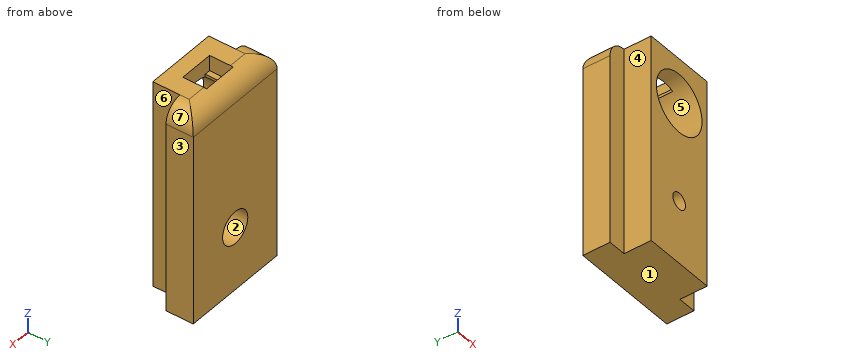
from build123d import *

# Parameters (mm, degrees)
SKETCH1_W           = 12
SKETCH1_H           = 23
BOSS_EXTRUDE1_DEPTH = 6
SKETCH2_W           = 2
SKETCH2_H           = 3
CUT_EXTRUDE1_DEPTH  = 25.515301344
SKETCH3_W           = 3.82
SKETCH3_H           = 2.6
CUT_EXTRUDE2_DEPTH  = 1.71
SKETCH4_W           = 2.566615902
SKETCH4_H           = 2.2
CUT_EXTRUDE3_DEPTH  = 3.1
CUT_EXTRUDE4_REACH  = 16.292
SKETCH5_R           = 3.265
FILLET1_R           = 2


with BuildPart() as part:
    # Sketch1 → Boss-Extrude1 (new body)
    with BuildSketch(Plane(origin=(0, 0, 0), x_dir=(1, 0, 0), z_dir=(0, 1, 0))):
        Rectangle(SKETCH1_W, SKETCH1_H)
    extrude(amount=BOSS_EXTRUDE1_DEPTH)

    # Sketch2 → Cut-Extrude1 (cut, through all)
    with BuildSketch(Plane.XY.offset(11.5)):
        with Locations((5, 1.5)):
            Rectangle(SKETCH2_W, SKETCH2_H)
        with Locations((-5, 1.5)):
            Rectangle(SKETCH2_W, SKETCH2_H)
    extrude(amount=-CUT_EXTRUDE1_DEPTH, mode=Mode.SUBTRACT)

    # Sketch3 → Cut-Extrude2 (cut)
    with BuildSketch(Plane.XY.offset(11.5)):
        with Locations((0, 3)):
            Rectangle(SKETCH3_W, SKETCH3_H)
    extrude(amount=-CUT_EXTRUDE2_DEPTH, mode=Mode.SUBTRACT)

    # Sketch4 → Cut-Extrude3 (cut)
    with BuildSketch(Plane.XY.offset(9.79)):
        with Locations((0, 2.8)):
            Rectangle(SKETCH4_W, SKETCH4_H)
    extrude(amount=-CUT_EXTRUDE3_DEPTH, mode=Mode.SUBTRACT)

    # Cut-Extrude4: up to this face of the body (flat: up to its plane)
    cut_extrude4_end = Plane(part.part.faces().sort_by_distance((0, 3.9, 8.24))[0])
    # Sketch5 → Cut-Extrude4 (cut, up to the picked face)
    with BuildSketch(Plane.XZ, mode=Mode.PRIVATE) as cut_extrude4_sk1:
        with Locations(Location((0, 6.5, 0), (0, 0, 270))):
            Circle(SKETCH5_R)
    cut_extrude4_tool1 = split(extrude(cut_extrude4_sk1.sketch, amount=-CUT_EXTRUDE4_REACH, mode=Mode.PRIVATE), bisect_by=cut_extrude4_end, keep=Keep.BOTH, mode=Mode.PRIVATE)
    add(cut_extrude4_tool1.solids().sort_by(Axis((0, 0, 6.5), (0, 1, 0)))[0], mode=Mode.SUBTRACT)

    # Fillet1
    # the kernel refuses this fillet: 2 mm, written as the material it takes off along each edge
    with BuildSketch(Plane(origin=(6, -2, 11.5), x_dir=(0, 0, -1), z_dir=(0, 1, 0))) as fillet1_piece_1:
        with BuildLine():
            CenterArc((FILLET1_R, FILLET1_R), FILLET1_R, 180, 90)
            Line((0, FILLET1_R), (0, 0))
            Line((0, 0), (FILLET1_R, 0))
        make_face()
    extrude(amount=13, mode=Mode.SUBTRACT)
    with BuildSketch(Plane(origin=(-11, 6, 11.5), x_dir=(0, 0, -1), z_dir=(1, 0, 0))) as fillet1_piece_2:
        with BuildLine():
            CenterArc((FILLET1_R, -FILLET1_R), FILLET1_R, 90, 90)
            Line((0, -FILLET1_R), (0, 0))
            Line((0, 0), (FILLET1_R, 0))
        make_face()
    extrude(amount=22, mode=Mode.SUBTRACT)
    with BuildSketch(Plane(origin=(-6, -2, 11.5), x_dir=(0, 0, -1), z_dir=(0, 1, 0))) as fillet1_piece_3:
        with BuildLine():
            CenterArc((FILLET1_R, -FILLET1_R), FILLET1_R, 90, 90)
            Line((0, -FILLET1_R), (0, 0))
            Line((0, 0), (FILLET1_R, 0))
        make_face()
    extrude(amount=13, mode=Mode.SUBTRACT)

    # Sketch7 → CSK SLOT for M1.6 Countersunk Flat Head Screw1 (revolve, cut)
    with BuildSketch(Plane(origin=(0, 6, -4.5), x_dir=(0, 0, 1), z_dir=(1, 0, 0))):
        Polygon((0, 0), (0, 6), (0.9, 6), (0.9, 4.9), (1.8, 4), (1.8, 0), align=None)
    revolve(axis=Axis((0, 12.35, -4.5), (0, -1, 0)), mode=Mode.SUBTRACT)


solid = part.part
Part model, mm, in its own coordinate system. Face numbers are marked on the shaded views. A direction names the side the tool comes from. Give positions to 0.01 mm unless a question says otherwise; leave off trailing zeros. Write each loop counter-clockwise with the first axis right and the second up, starting at its lowest first coordinate (ties: lowest second). Pieces come first, ordered by that corner, then holes.
1) Cut at A-A on z = -4.5. Write the cut outline in (x, y).
Resolved:
outline: (-6, 3) - (-4, 3) - (-4, 0) - (-0.9, 0) - (-0.9, 1.1) - (-1.8, 2) - (-1.8, 6) - (-6, 6) - close; (0.9, 0) - (4, 0) - (4, 3) - (6, 3) - (6, 6) - (1.8, 6) - (1.8, 2) - (0.9, 1.1) - close
2) Cut at B-B on x = 0. Write the cut outline in (y, z) (3 decimals), then the cut area to 3 significant figures.
Resolved:
outline: (0, -11.5) - (6, -11.5) - (6, -6.3) - (2, -6.3) - (1.1, -5.4) - (0, -5.4) - close; (0, -3.6) - (1.1, -3.6) - (2, -2.7) - (6, -2.7) - (6, 9.5) arc R2 ccw to (4.3, 11.477) - (4.3, 9.79) - (3.9, 9.79) - (3.9, 3.235) - (0, 3.235) - close; (0, 9.765) - (1.7, 9.765) - (1.7, 11.5) - (0, 11.5) - close
area: 88.4 mm2
3) Cut at D-D on y = 1.4. Write the cut outline in (x, z) (3 decimals).
Resolved:
outline: (-4, -11.5) - (4, -11.5) - (4, 11.5) - (-4, 11.5) - close; hole circle Ø6.53 at (0, 6.5); hole circle Ø2.4 at (0, -4.5)
4) Which spindle directions (+Z, -Z, +X, -X, +Y, -Y) get a long thin tool onto all of the face, cutting with end or side? Do the marked faces 4, 5, 6 and 7. Say none if no direction does.
Resolved:
face 4: +Z, -Z, -X, -Y
face 5: -Y
face 6: +Z, -Z, +X, -Y
face 7: +Z, +X, +Y, -Y
5) Pin check, flat tips, straight feed: pin 1 (0.5 mm diameter, centred on y = 2.5, z = 10.5, fed in from +X); pin 2 (1.4 mm diameter, centred on y = 3.5, z = 10.5, fed in from -X); pin 3 (0.6 mm diameter, centred on x = 0.5, z = 11, fed in from +Y). Stop position of each tip, or through.
Resolved:
pin 1: stops at x = 4
pin 2: stops at x = -5.98
pin 3: stops at y = 5.6
6) Probe L1, parallel to X at y = 2.9, z = 6.5 (3 decimals); L2, parallel to Z at x = 0, y = 0.4 (3 decimals); L3, parallel to Z at x = 0, y = 4.1. List the from-to ranges inside material, lowest first.
Resolved:
L1: x = -4 to -3.265, 3.265 to 4
L2: z = -11.5 to -5.4, -3.6 to 3.235, 9.765 to 11.5
L3: z = -11.5 to -6.3, -2.7 to 9.79
7) Cut at C-C on y = 5.3. Write the cut outline in (x, z).
Resolved:
outline: (-6, -11.5) - (6, -11.5) - (6, 9.5) arc R2 ccw to (5.3, 11.02) - (-5.3, 11.02) arc R2 ccw to (-6, 9.5) - close; hole circle Ø3.6 at (0, -4.5)
8) Two-plate mould, pull along Z, no slides. Class the marked faces 1, 2 and 3: released by +Z, released by -Z, zero draft, split by the parting line, or undercut.
Resolved:
face 1: released by -Z
face 2: undercut
face 3: zero draft
